Part model, mm, in its own coordinate system. Face numbers are marked on the shaded views. A direction names the side the tool comes from. Coordinates: 2 decimals unless noted, no trailing zeros. Loops run counter-clockwise (first coordinate to the right, second up) from the corner with the lowest first, then second, coordinate; pieces in that order, holes last. Notation, with made-up numbers: M 33.25,45 L 53.25,45 A13 ccw 53.25,60 Z; hole C 53.5,11 d2. An arc over 180 degrees is marked long. Use a Markdown table: item, result. Add a question column.
1) Pin check, flat tips, straight feed: pin 1 Ø4 at (x, z) = (15.68, -17.4) entering from +Y; pin 2 Ø5 at (y, z) = (-26, -3) entering from +X; pin 3 Ø5 at (y, z) = (-12.5, -5.5) entering from -X. Stop position of each tip, or through.
2) Tool access for the marked faces 1, 2, 3 and 4: list every direction of +Z, -Z, +X, -X, +Y, -Y with a clear straight run to the whole face (end or side of a thin tool).
3) Wall check: probe 1 along X at (y, z) = (-16, -4.5); probe 2 along Y at (x, z) = (-26, 2); probe 3 along Z at (x, y) = (-3.5, -63) (3 decimals). Give the ranges that are in metal, low to high. Write a range as from..to.
4) Band-saw the part on B-B (y = -71.5). List the corners of the cut face in (x, z) (3 decimals), plus the area to 3 significant figures.
from build123d import *

# Parameters (mm, degrees)
F1_DEPTH = 6.35
F2_W     = 49.21945557
F2_H     = 19.05
F3_DEPTH = 81.28
F4_W     = 49.21945557
F4_H     = 19.05
F4_R     = 1.524
F5_DEPTH = 5.588
F6_R     = 2.54


with BuildPart() as f1:
    # F0 (on Front) → F1 (new body)
    with BuildSketch(Plane.XZ):
        with BuildLine():
            ThreePointArc((-27.178, 9.525), (-36.703, 0), (-27.178, -9.525))
            Line((-27.178, -9.525), (-27.178, -1.397))
            ThreePointArc((-27.178, -1.397), (-28.575, 0), (-27.178, 1.397))
            Line((-27.178, 1.397), (-27.178, 9.525))
        make_face()
        with BuildLine():
            Line((-27.178, -9.525), (27.178, -9.525))
            Line((27.178, -9.525), (27.178, -1.397))
            ThreePointArc((27.178, -1.397), (25.781, 0), (27.178, 1.397))
            Line((27.178, 1.397), (27.178, 9.525))
            Line((27.178, 9.525), (-27.178, 9.525))
            Line((-27.178, 9.525), (-27.178, 1.397))
            ThreePointArc((-27.178, 1.397), (-26.1901718267, 0.9878281733), (-25.781, 0))
            ThreePointArc((-25.781, 0), (-26.1901718267, -0.9878281733), (-27.178, -1.397))
            Line((-27.178, -1.397), (-27.178, -9.525))
        make_face()
        with BuildLine():
            Line((27.178, -1.397), (27.178, -9.525))
            ThreePointArc((27.178, -9.525), (36.703, 0), (27.178, 9.525))
            Line((27.178, 9.525), (27.178, 1.397))
            ThreePointArc((27.178, 1.397), (28.1658281733, 0.9878281733), (28.575, 0))
            ThreePointArc((28.575, 0), (28.1658281733, -0.9878281733), (27.178, -1.397))
        make_face()
    extrude(amount=F1_DEPTH)

    # F2 (on face) → F3 (join)
    with BuildSketch(Plane.XZ.offset(6.35)):
        Rectangle(F2_W, F2_H)
    extrude(amount=F3_DEPTH)

    # F4 (on face) → F5 (join)
    with BuildSketch(Plane.XZ.offset(87.63)):
        Rectangle(F4_W, F4_H)
        Polygon((24.6470458806, 9.525), (24.609727785, 9.525), (24.609727785, -9.525), (-24.609727785, -9.525), (-24.609727785, -22.733), (24.6470458806, -22.733), align=None)
        with Locations((-15.678541685, -17.399)):
            Circle(F4_R, mode=Mode.SUBTRACT)
        with Locations((15.678541685, -17.399)):
            Circle(F4_R, mode=Mode.SUBTRACT)
    extrude(amount=F5_DEPTH)

    # F6
    f6_edges = [f1.edges().sort_by_distance(p)[0] for p in [
        (-24.609728, -90.424, -22.733),
        (24.647046, -90.424, -22.733),
    ]]
    fillet(f6_edges, radius=F6_R)


solid = f1.part
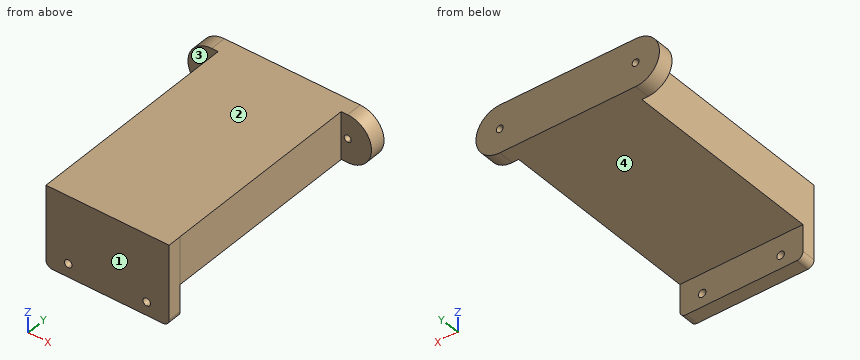
Entries:
| question | item | result |
|---|---|---|
| 1 | pin 1 | y = -87.63 |
| 1 | pin 2 | x = 24.61 |
| 1 | pin 3 | x = -24.61 |
| 2 | face 1 | +Z, -Z, +X, -X, -Y |
| 2 | face 2 | +Z, +X, -X, +Y, -Y |
| 2 | face 3 | +Z, -Z, -X, -Y |
| 2 | face 4 | -Z, +X, -X, +Y |
| 3 | probe 1 | -24.61..24.61 |
| 3 | probe 2 | -6.35..0 |
| 3 | probe 3 | -9.525..9.525 |
| 4 | outline | M -24.61,-9.525 L 24.61,-9.525 L 24.61,9.525 L -24.61,9.525 Z |
| 4 | area | 938 mm2 |
